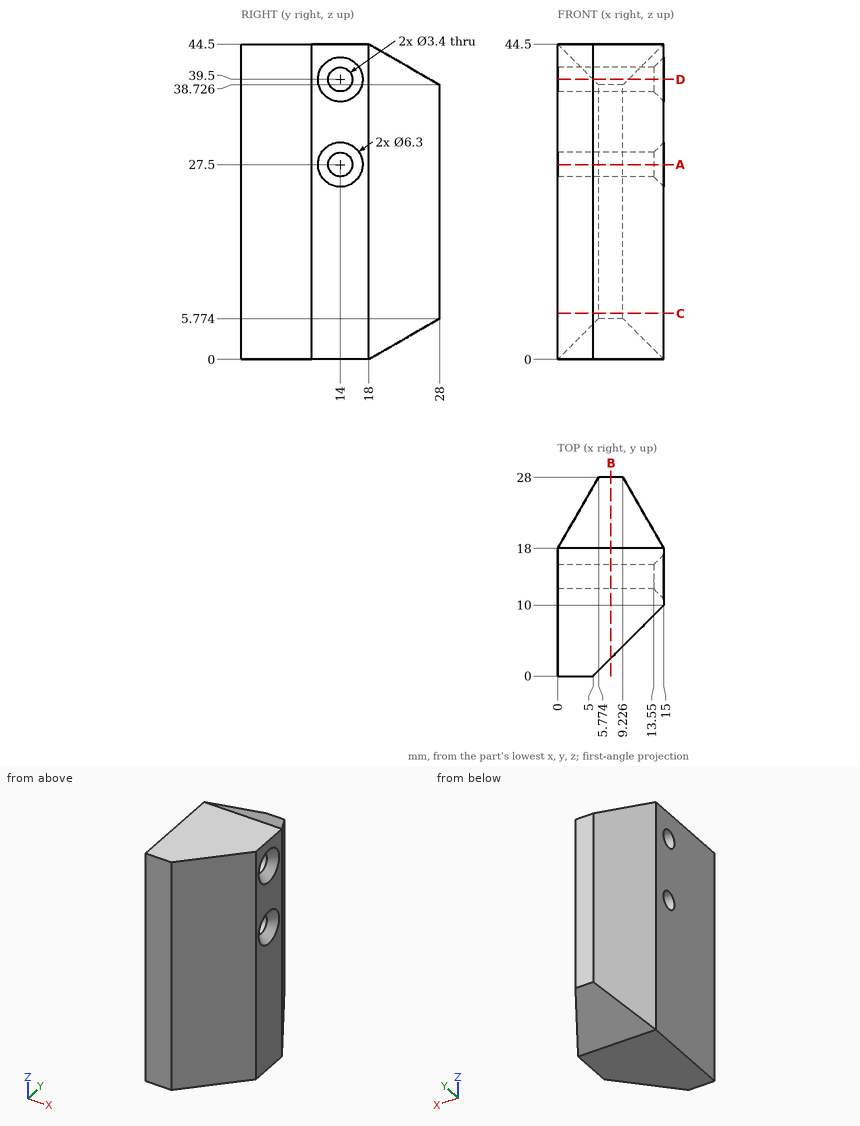
Drawing for the job (mm, zero at the part's lowest x, y, z). Round coordinates to 2 decimals unless told otherwise and drop trailing zeros. Order: outer loops, then holes, each group sorted by start corner. A loop starts at its lowest first (then second) coordinate and runs counter-clockwise, first axis right, second up. Notation, with made-up numbers: (-36, -11.75) -> (-13, -11.75) arc R22 ccw to (-13, 12.25) -> close; hole circle Ø1 at (-35, 17.25). An arc over 180 degrees is marked (long way). Write item = value, one per line. Start each with the question number.
(1) Cut at D-D, the plane z = 39.5. List the corners of the cut face in (x, y).
(2) Probe line 1 (Z direction, x = 6.75, y = 14); line 2 (Z direction, x = 6.5, y = 12.5); line 3 (Y direction, x = 6, z = 39.5). List the from-to ranges inside material, lowest first. Write a range as [from, to].
(3) Cut at B-B, the plane x = 7.5. List the corners of the cut face in (y, z).
(4) Cut at A-A, the plane z = 27.5. List the corners of the cut face in (x, y).
(5) Pin check, flat tips, straight feed: P1, Ø6, axis at x = 12, z = 23, coming from the +Y side; P2, Ø8, axis at x = 6, y = 24, coming from the +Z side (1 decimal); P3, Ø1.5, axis at y = 3, z = 11, coming from the +X side; P4, Ø5.5, axis at y = 14, z = 27.5, coming from the +X side. Stop position of each tip, or through.
(6) Cut at C-C, the plane z = 6.5. List the corners of the cut face in (x, y).
Model answer:
q1.outline = (0, 0) -> (5, 0) -> (15, 10) -> (15, 10.85) -> (13.55, 12.3) -> (0, 12.3) -> close; (0, 15.7) -> (13.55, 15.7) -> (15, 17.15) -> (15, 18) -> (10, 26.66) -> (5, 26.66) -> (0, 18) -> close
q2.line_1 = [0, 25.8], [29.2, 37.8], [41.2, 44.5]
q2.line_2 = [0, 26.7], [28.3, 38.7], [40.3, 44.5]
q2.line_3 = [1, 12.3], [15.7, 26.66]
q3.outline = (2.5, 0) -> (18, 0) -> (28, 5.77) -> (28, 38.73) -> (18, 44.5) -> (2.5, 44.5) -> close; hole circle Ø3.4 at (14, 27.5); hole circle Ø3.4 at (14, 39.5)
q4.outline = (0, 0) -> (5, 0) -> (15, 10) -> (15, 10.85) -> (13.55, 12.3) -> (0, 12.3) -> close; (0, 15.7) -> (13.55, 15.7) -> (15, 17.15) -> (15, 18) -> (9.23, 28) -> (5.77, 28) -> (0, 18) -> close
q5.P1 = 28
q5.P2 = 43.3
q5.P3 = 8.75
q5.P4 = 14.6
q6.outline = (0, 0) -> (5, 0) -> (15, 10) -> (15, 18) -> (9.23, 28) -> (5.77, 28) -> (0, 18) -> close
